```python
from build123d import *

# Parameters (mm, degrees)
BOSS_EXTRUDE1_DEPTH     = 2.54
SKETCH2_R               = 2
CUT_EXTRUDE1_DEPTH      = 1
CUT_EXTRUDE1_DEPTH_BACK = 3.54


with BuildPart() as part:
    # Sketch1 → Boss-Extrude1 (new body)
    with BuildSketch(Plane(origin=(0, 0, 0), x_dir=(1, 0, 0), z_dir=(0, 1, 0))):
        with BuildLine():
            Line((-89.636017598, 11), (-11.963982402, 11))
            ThreePointArc((-11.963982402, 11), (0, 16.252288298), (11.963982402, 11))
            Line((11.963982402, 11), (89.636017598, 11))
            ThreePointArc((89.636017598, 11), (117.852288298, 0), (89.636017598, -11))
            Line((89.636017598, -11), (11.963982402, -11))
            ThreePointArc((11.963982402, -11), (0, -16.252288298), (-11.963982402, -11))
            Line((-11.963982402, -11), (-89.636017598, -11))
            ThreePointArc((-89.636017598, -11), (-117.852288298, 0), (-89.636017598, 11))
        make_face()
    extrude(amount=BOSS_EXTRUDE1_DEPTH)

    # Sketch2 → Cut-Extrude1 (cut, two sides)
    with BuildSketch(Plane(origin=(0, 2.54, 0), x_dir=(1, 0, 0), z_dir=(0, 1, 0))) as cut_extrude1_sk:
        with Locations((-101.6, 0)):
            Circle(SKETCH2_R)
        with Locations((101.6, 0)):
            Circle(SKETCH2_R)
        Circle(SKETCH2_R)
    extrude(amount=CUT_EXTRUDE1_DEPTH, mode=Mode.SUBTRACT)
    extrude(cut_extrude1_sk.sketch, amount=-CUT_EXTRUDE1_DEPTH_BACK, mode=Mode.SUBTRACT)


solid = part.part
```
Input: part model. Units: mm. Frame: model coordinates. Give positions to 0.01 mm unless a question says otherwise; leave off trailing zeros. Order: outer loops, then holes, each group sorted by start corner. A loop starts at its lowest first (then second) coordinate and runs counter-clockwise, first axis right, second up.
1. Section C-C on y = 0.75. Return the cut outline in (x, z), and give its area (3 significant figures).
Derived:
outline: (-89.64, -11) - (-11.96, -11) arc R16.25 ccw to (11.96, -11) - (89.64, -11) arc R16.25 ccw (long way) to (89.64, 11) - (11.96, 11) arc R16.25 ccw to (-11.96, 11) - (-89.64, 11) arc R16.25 ccw (long way) to start; hole circle Ø4 at (-101.6, 0); hole circle Ø4 at (0, 0); hole circle Ø4 at (101.6, 0)
area: 5,610 mm2
2. Mould query, pull axis Z, two halves, no side actions, for faces 1 (the cylindrical face through (0, 1, 2)), 2 (the cylindrical face through (-117.843, 1.252, 0.546)), 3 (the flat face through (2, 2.54, 3)). Classes: released by +Z, released by -Z, zero draft, split by the parting line, or undercut.
Derived:
face 1: undercut
face 2: split by the parting line
face 3: zero draft
3. Material intervals for L1, parallel to Z at x = -101.6, y = 0.95; L2, parallel to X at y = 0.55, z = 13; L3, parallel to Z at x = -38, y = 0.7, sorted ascending.
Derived:
L1: z = -16.25 to -2, 2 to 16.25
L2: x = -111.35 to -91.85, -9.75 to 9.75, 91.85 to 111.35
L3: z = -11 to 11
4. Section A-A on x = -101.6. Return the cut outline in (y, z).
Derived:
outline: (0, -16.25) - (2.54, -16.25) - (2.54, -2) - (0, -2) - close; (0, 2) - (2.54, 2) - (2.54, 16.25) - (0, 16.25) - close
5. Section B-B on z = 0. Return the cut outline in (x, y), and give its area (3 significant figures).
Derived:
outline: (-117.85, 0) - (-103.6, 0) - (-103.6, 2.54) - (-117.85, 2.54) - close; (-99.6, 0) - (-2, 0) - (-2, 2.54) - (-99.6, 2.54) - close; (2, 0) - (99.6, 0) - (99.6, 2.54) - (2, 2.54) - close; (103.6, 0) - (117.85, 0) - (117.85, 2.54) - (103.6, 2.54) - close
area: 568 mm2
6. Section D-D on z = -13. Return the cut outline in (x, y).
Derived:
outline: (-111.35, 0) - (-91.85, 0) - (-91.85, 2.54) - (-111.35, 2.54) - close; (-9.75, 0) - (9.75, 0) - (9.75, 2.54) - (-9.75, 2.54) - close; (91.85, 0) - (111.35, 0) - (111.35, 2.54) - (91.85, 2.54) - close
7. Pin query (flat end, axial travel): pin 1 (3.5 mm diameter, centred on x = 0, z = 0, fed in from -Y); pin 2 (1.3 mm diameter, centred on x = -54, y = 1.5, fed in from -Z); pin 3 (1 mm diameter, centred on x = -12, y = 0.5, fed in from -Z); pin 4 (0.8 mm diameter, centred on x = -64.5, y = 1, fed in from +Z). Return the tip coordinate at first contact, or that it passes through.
Derived:
pin 1: passes through
pin 2: stops at z = -11
pin 3: stops at z = -11.48
pin 4: stops at z = 11
